Could you check a few things on this model? Use its own coordinates, in mm. A direction names the side the tool comes from. Round coordinates to 2 decimals unless told otherwise and drop trailing zeros. Write each loop counter-clockwise with the first axis right and the second up, starting at its lowest first coordinate (ties: lowest second). Pieces come first, ordered by that corner, then holes. Notation, with made-up numbers: (29.25, -28) -> (60.25, -28) arc R7 ccw to (60.25, -19) -> close; hole circle Ø10 at (72, 34). An arc over 180 degrees is marked (long way). Answer as CSV lines item,"result". Start each with the question number.
Q1. Imagine slicing it at D-D on y = 8. Give the number of separate pieces and of enclosed holes in the cut face, and give its area (3 significant figures).
Q2. Imagine slicing it at A-A on x = 0. Please give me the cut outline in (y, z), and give its area (3 significant figures).
Q3. Imagine slicing it at C-C on z = -27.5. Please give me the cut outline in (x, y).
Q4. Imagine slicing it at B-B on y = 18.75. Please give me the cut outline in (x, z), and give its area (3 significant figures).
Q5. Will these pins go through, and if not, where does the flat tip stop? pin 1 Ø12 at (y, z) = (7, 12) entering from -X; pin 2 Ø5 at (x, z) = (-2.5, -27) entering from +Y; pin 3 Ø10 at (y, z) = (8, 59) entering from -X.
Q6. If we mould it in two halves opening along X, with no side actions, what happens to faces 1 (the flat face through (-20, 7, 15)), 2 (the flat face through (12, 10, 23)), 3 (the flat face through (-22, 7, -24))? For each: pulls with the +X half, pulls with the -X half, needs draft (parallel to the pull), parting line crosses it, or undercut.
Q7. For faces 4 (the flat face through (4, 13, -20)), 5 (the cylindrical face through (-20, 4, -10)), 6 (the flat face through (-20, 15, -23)), 7 (the flat face through (7.5, 2, 74)), which set-ups out of +Z, -Z, +X, -X, +Y, -Y let a thin tool reach every point of the face, with its end or its side?
Q8. If I drill on line 1 (X direction, y = 12.15, z = -27.5); line 2 (Y direction, x = 8.5, z = 0); line 3 (Y direction, x = -5.5, z = -21.5), over which ranges is the centre line in solid material (lowest first)? Write a range as [from, to].
from build123d import *

# Parameters (mm, degrees)
SKETCH1_W            = 40
SKETCH1_H            = 50
BOSS_EXTRUDE1_DEPTH  = 5
SKETCH3_W            = 5
SKETCH3_H            = 5
BOSS_EXTRUDE5_DEPTH  = 20
SKETCH3_3_W          = 15
SKETCH3_3_H          = 5
SKETCH3_3_W_2        = 5
BOSS_EXTRUDE6_DEPTH  = 10
CUT_EXTRUDE3_DEPTH   = 4
BOSS_EXTRUDE9_START  = 3
BOSS_EXTRUDE9_DEPTH  = 3
SKETCH12_W           = 5
SKETCH12_H           = 5
BOSS_EXTRUDE10_DEPTH = 5
SKETCH13_R           = 1.5
CUT_EXTRUDE4_DEPTH   = 5
SKETCH14_W           = 15
SKETCH14_H           = 5
BOSS_EXTRUDE11_DEPTH = 80
SKETCH15_W           = 15
SKETCH15_H           = 20
BOSS_EXTRUDE13_DEPTH = 20
CUT_EXTRUDE7_DEPTH   = 15


with BuildPart() as part:
    # Sketch1 → Boss-Extrude1 (new body)
    with BuildSketch(Plane(origin=(0, 0, 0), x_dir=(1, 0, 0), z_dir=(0, 1, 0))):
        Rectangle(SKETCH1_W, SKETCH1_H)
    extrude(amount=BOSS_EXTRUDE1_DEPTH)

    # Sketch3 → Boss-Extrude5 (add)
    with BuildSketch(Plane(origin=(0, 5, 0), x_dir=(1, 0, 0), z_dir=(0, 1, 0))):
        with Locations((17.5, -22.5)):
            Rectangle(SKETCH3_W, SKETCH3_H)
        with Locations((9.5, 22.5)):
            Rectangle(SKETCH3_W, SKETCH3_H)
    extrude(amount=BOSS_EXTRUDE5_DEPTH)

    # Sketch3_3 → Boss-Extrude6 (add)
    with BuildSketch(Plane(origin=(0, 5, 0), x_dir=(1, 0, 0), z_dir=(0, 1, 0))):
        with Locations((-0.5, 22.5)):
            Rectangle(SKETCH3_3_W, SKETCH3_3_H)
        Polygon((-16, -20), (-16, 25), (-20, 25), (-20, -25), (7, -25), (7, -20), align=None)
        with Locations((17.5, 22.5)):
            Rectangle(SKETCH3_3_W_2, SKETCH3_3_H)
        with Locations((9.5, -22.5)):
            Rectangle(SKETCH3_3_W_2, SKETCH3_3_H)
    extrude(amount=BOSS_EXTRUDE6_DEPTH)

    # Sketch8 → Cut-Extrude3 (cut)
    with BuildSketch(Plane.ZY.offset(20)):
        with BuildLine():
            Line((1, 15), (-21, 15))
            ThreePointArc((-21, 15), (-10, 4), (1, 15))
        make_face()
    extrude(amount=-CUT_EXTRUDE3_DEPTH, mode=Mode.SUBTRACT)

    # Sketch10 → Boss-Extrude9 (add)
    with BuildSketch(Plane.ZY.offset(20).offset(BOSS_EXTRUDE9_START)):
        with BuildLine():
            Line((1, 15), (4, 15))
            Line((4, 15), (4, 0))
            Line((4, 0), (-24, 0))
            Line((-24, 0), (-24, 15))
            Line((-24, 15), (-21, 15))
            ThreePointArc((-21, 15), (-10, 4), (1, 15))
        make_face()
    extrude(amount=-BOSS_EXTRUDE9_DEPTH)

    # Sketch12 → Boss-Extrude10 (add)
    with BuildSketch(Plane(origin=(0, 0, -25), x_dir=(-1, 0, 0), z_dir=(0, 0, -1))):
        with Locations((0, 12.5)):
            Rectangle(SKETCH12_W, SKETCH12_H)
    extrude(amount=BOSS_EXTRUDE10_DEPTH)

    # Sketch13 → Cut-Extrude4 (cut)
    with BuildSketch(Plane.XZ.offset(-10)):
        with Locations(Location((0, -27.5, 0), (0, 0, 270))):
            Circle(SKETCH13_R)
    extrude(amount=-CUT_EXTRUDE4_DEPTH, mode=Mode.SUBTRACT)

    # Sketch14 → Boss-Extrude11 (add)
    with BuildSketch(Plane.XY.offset(25)):
        with Locations((0, 2.5)):
            Rectangle(SKETCH14_W, SKETCH14_H)
    extrude(amount=BOSS_EXTRUDE11_DEPTH)

    # Sketch15 → Boss-Extrude13 (add)
    with BuildSketch(Plane(origin=(0, 5, 0), x_dir=(1, 0, 0), z_dir=(0, 1, 0))):
        with Locations((0, -95)):
            Rectangle(SKETCH15_W, SKETCH15_H)
    extrude(amount=BOSS_EXTRUDE13_DEPTH)

    # Sketch18 → Cut-Extrude7 (cut)
    with BuildSketch(Plane.ZY.offset(7.5)):
        Polygon((105, 0), (90.56624327, 25), (105, 25), align=None)
    extrude(amount=-CUT_EXTRUDE7_DEPTH, mode=Mode.SUBTRACT)


solid = part.part
Checks:
1,separate pieces,"6"
1,enclosed holes,"0"
1,area,"686 mm^2"
2,outline,"(0, -25) -> (10, -25) -> (10, -26) -> (15, -26) -> (15, -20) -> (5, -20) -> (5, 20) -> (15, 20) -> (15, 25) -> (5, 25) -> (5, 85) -> (25, 85) -> (25, 90.57) -> (0, 105) -> close; (10, -30) -> (15, -30) -> (15, -29) -> (10, -29) -> close"
2,area,"980 mm^2"
3,outline,"(-2.5, 10) -> (-1.5, 10) -> (-1.5, 15) -> (-2.5, 15) -> close; (1.5, 10) -> (2.5, 10) -> (2.5, 15) -> (1.5, 15) -> close"
4,outline,"(-7.5, 85) -> (7.5, 85) -> (7.5, 94.17) -> (-7.5, 94.17) -> close; (7, -25) -> (12, -25) -> (12, -20) -> (7, -20) -> close; (15, 20) -> (20, 20) -> (20, 25) -> (15, 25) -> close"
4,area,"188 mm^2"
5,pin 1,"x = -20"
5,pin 2,"y = 15"
5,pin 3,"x = -7.5"
6,face 1,"pulls with the -X half"
6,face 2,"undercut"
6,face 3,"needs draft"
7,face 4,"+X, +Y"
7,face 5,"-X, +Y"
7,face 6,"+Z, -Z, -X, +Y"
7,face 7,"+Z, +X, +Y, -Y"
8,line 1,"[-2.5, -1.5], [1.5, 2.5]"
8,line 2,"[0, 5]"
8,line 3,"[0, 15]"
